The listing builds one solid part. Answer for the finished solid, in the listing's coordinates (mm). A direction names the side the tool comes from. Coordinates: 2 decimals unless noted, no trailing zeros. Order: outer loops, then holes, each group sorted by start corner. A loop starts at its lowest first (then second) coordinate and runs counter-clockwise, first axis right, second up. Notation, with made-up numbers: (62.5, 51) - (86.5, 51) arc R15 cw to (86.5, 75) - close; hole circle Ø10 at (-14.75, 36.5). An arc over 180 degrees is marked (long way). Use a Markdown table: item, result. Add a question column.
Item 1: The part is cut by section B-B, the plane y = 25. Give the vertices of the cut face in (x, z).
Item 2: For faces 5 (the flat face through (-11, 25, 48)), 6 (the flat face through (0, -20.77, 56)), 7 (the flat face through (0, 24, 52.664)), determine the directions among +Z, -Z, +X, -X, +Y, -Y from which every point of the face is accessible in a straight line to the end or side of a thin tool.
Item 3: The part is cut by section D-D, the plane z = 36. Give the vertices of the cut face in (x, y).
Item 4: Find the intervals of material crossed by line 1 along Y through (x, z) = (-8.5, 23.5); line 2 along Y through (x, z) = (9, 42); line 3 along Z through (x, y) = (7, -11), in increasing order.
Item 5: The part is cut by section A-A, the plane z = 24. Give the vertices of the cut face in (x, y).
Item 6: The mould has two halves that part along Y. Classify faces 1 (the flat face through (0, 30.77, 29)), 2 (the flat face through (0, -23, 52.664)), 3 (the flat face through (0, -26, 59)), 4 (the flat face through (0, -30.77, 29)): released by +Y, released by -Y, zero draft, split by the parting line, or undercut.
Item 7: Flat-ended cylindrical pins translate along their axes: P1, Ø2.5, axis at y = 25.5, z = 48, coming from the -X side; P2, Ø4, axis at x = -6, y = -23.5, coming from the -Z side; P3, Ø12, axis at x = -1, y = -0.5, coming from the +Z side; P4, Ø5, axis at y = 6, z = 13, coming from the -X side. Find the tip coordinate at first contact, or state that the pin passes through.
from build123d import *

# Parameters (mm, degrees)
ESBO_O1_W                  = 30
ESBO_O1_H                  = 10
RESSALTO_EXTRUS_O1_DEPTH   = 59
RESSALTO_EXTRUS_O1_2_DEPTH = 59
ESBO_O2_W                  = 30
ESBO_O2_H                  = 41.54
RESSALTO_EXTRUS_O2_DEPTH   = 10
CORTE_EXTRUS_O1_DEPTH      = 73.991731724
CORTE_EXTRUS_O2_DEPTH      = 4


with BuildPart() as part:
    # Esbo_o1 → Ressalto-extrus_o1 (new body)
    with BuildSketch(Plane.XY):
        with Locations((0, 25.77)):
            Rectangle(ESBO_O1_W, ESBO_O1_H)
    extrude(amount=RESSALTO_EXTRUS_O1_DEPTH)



with BuildPart() as body_2:
    # Esbo_o1 → Ressalto-extrus_o1 2 (new body)
    with BuildSketch(Plane.XY):
        with Locations((0, -25.77)):
            Rectangle(ESBO_O1_W, ESBO_O1_H)
    extrude(amount=RESSALTO_EXTRUS_O1_2_DEPTH)


with BuildPart() as part_1:
    add(part.part)

    add(body_2.part)  # Ressalto-extrus_o2 merges body 2
    # Esbo_o2 → Ressalto-extrus_o2 (add)
    with BuildSketch(Plane(origin=(0, 0, 0), x_dir=(-1, 0, 0), z_dir=(0, 0, -1))):
        Rectangle(ESBO_O2_W, ESBO_O2_H)
    extrude(amount=-RESSALTO_EXTRUS_O2_DEPTH)

    # Esbo_o3 → Corte-extrus_o1 (cut, through all)
    with BuildSketch(Plane.ZY.offset(15)):
        with BuildLine():
            ThreePointArc((51.8897547, -26.423845407), (52.437454615, -26.196980674), (52.664319348, -25.649280759))
            Line((52.664319348, -25.649280759), (52.664319348, -20.77))
            Line((52.664319348, -20.77), (52.564319348, -20.77))
            Line((52.564319348, -20.77), (34.5, -20.77))
            Line((34.5, -20.77), (34.464319348, -20.770417185))
            Line((34.464319348, -20.770417185), (34.464319348, -25.649280759))
            ThreePointArc((34.464319348, -25.649280759), (34.69118408, -26.196980674), (35.238883995, -26.423845407))
            Line((35.238883995, -26.423845407), (37.994984805, -26.423845407))
            Line((37.994984805, -26.423845407), (38.294984805, -26.423845407))
            Line((38.294984805, -26.423845407), (38.294984805, -25.584623249))
            ThreePointArc((38.294984805, -25.584623249), (39.064319348, -21.220238146), (39.83365389, -25.584623249))
            Line((39.83365389, -25.584623249), (39.83365389, -26.423845407))
            Line((39.83365389, -26.423845407), (40.13365389, -26.423845407))
            Line((40.13365389, -26.423845407), (47.294984805, -26.423845407))
            Line((47.294984805, -26.423845407), (47.294984805, -25.584623249))
            ThreePointArc((47.294984805, -25.584623249), (48.064319348, -21.220238146), (48.83365389, -25.584623249))
            Line((48.83365389, -25.584623249), (48.83365389, -26.423845407))
            Line((48.83365389, -26.423845407), (49.215424515, -26.423845407))
            Line((49.215424515, -26.423845407), (51.8897547, -26.423845407))
        make_face()
        with BuildLine():
            Line((34.464319348, 27.162244637), (34.464319348, 20.77))
            Line((34.464319348, 20.77), (34.5, 20.77))
            Line((34.5, 20.77), (52.564319348, 20.77))
            Line((52.564319348, 20.77), (52.664319348, 20.77))
            Line((52.664319348, 20.77), (52.664319348, 27.13384671))
            ThreePointArc((52.664319348, 27.13384671), (52.473932816, 27.593480457), (52.014299068, 27.783866989))
            Line((52.014299068, 27.783866989), (48.83365389, 27.783866989))
            Line((48.83365389, 27.783866989), (48.853388433, 27.775806736))
            Line((48.853388433, 27.775806736), (48.83365389, 27.775908805))
            Line((48.83365389, 27.775908805), (48.83365389, 27.124623249))
            ThreePointArc((48.83365389, 27.124623249), (48.064319348, 22.760238146), (47.294984805, 27.124623249))
            Line((47.294984805, 27.124623249), (47.294984805, 27.783866989))
            Line((47.294984805, 27.783866989), (40.021105511, 27.821488377))
            Line((40.021105511, 27.821488377), (39.721105511, 27.821488377))
            Line((39.721105511, 27.821488377), (39.721105511, 27.162244637))
            ThreePointArc((39.721105511, 27.162244637), (39.064319348, 22.760238146), (38.407533184, 27.162244637))
            Line((38.407533184, 27.162244637), (38.407533184, 27.821488377))
            Line((38.407533184, 27.821488377), (38.107533184, 27.821488377))
            Line((38.107533184, 27.821488377), (35.104983392, 27.821488377))
            ThreePointArc((35.104983392, 27.821488377), (34.654639493, 27.631168232), (34.464319348, 27.180824333))
            Line((34.464319348, 27.180824333), (34.464319348, 27.162244637))
        make_face()
    extrude(amount=-CORTE_EXTRUS_O1_DEPTH, mode=Mode.SUBTRACT)

    # Esbo_o4 → Corte-extrus_o2 (cut)
    with BuildSketch(Plane.ZY.offset(15)):
        with BuildLine():
            Line((47.294984805, 27.783866989), (48.853388433, 27.775806736))
            Line((48.853388433, 27.775806736), (48.853388433, 27.117338044))
            ThreePointArc((48.853388433, 27.117338044), (48.055619332, 22.760254966), (47.291568671, 27.123377136))
            Line((47.291568671, 27.123377136), (47.294984805, 27.783866989))
        make_face()
        with BuildLine():
            Line((38.407533184, 27.821488377), (38.407533184, 27.162244637))
            ThreePointArc((38.407533184, 27.162244637), (39.064319348, 22.760238146), (39.721105511, 27.162244637))
            Line((39.721105511, 27.162244637), (39.721105511, 27.821488377))
            Line((39.721105511, 27.821488377), (38.407533184, 27.821488377))
        make_face()
    extrude(amount=-CORTE_EXTRUS_O2_DEPTH, mode=Mode.SUBTRACT)


solid = part_1.part
Solution:
| question | item | result |
|---|---|---|
| 1 | outline | (-15, 0) - (15, 0) - (15, 34.46) - (-15, 34.46) - close; (-15, 52.66) - (15, 52.66) - (15, 59) - (-15, 59) - close; (-11, 36.81) - (15, 36.81) - (15, 41.31) - (-11, 41.31) - close; (-11, 45.81) - (15, 45.81) - (15, 50.31) - (-11, 50.31) - close |
| 2 | face 5 | -X |
| 2 | face 6 | +Z, +X, -X |
| 2 | face 7 | +X, -X |
| 3 | outline | (-15, -30.77) - (15, -30.77) - (15, -26.42) - (-15, -26.42) - close; (-15, 27.82) - (15, 27.82) - (15, 30.77) - (-15, 30.77) - close |
| 4 | line 1 | y = -30.77 to -20.77, 20.77 to 30.77 |
| 4 | line 2 | y = -30.77 to -26.42, 27.81 to 30.77 |
| 4 | line 3 | z = 0 to 10 |
| 5 | outline | (-15, -30.77) - (15, -30.77) - (15, -20.77) - (-15, -20.77) - close; (-15, 20.77) - (15, 20.77) - (15, 30.77) - (-15, 30.77) - close |
| 6 | face 1 | released by +Y |
| 6 | face 2 | undercut |
| 6 | face 3 | zero draft |
| 6 | face 4 | released by -Y |
| 7 | P1 | stops at x = -11 |
| 7 | P2 | stops at z = 0 |
| 7 | P3 | stops at z = 10 |
| 7 | P4 | passes through |
